For this review, take the finished solid that the model builds, in its own axes (mm). A direction names the side the tool comes from. Give positions to 0.01 mm unless a question says otherwise; leave off trailing zeros. Write each loop counter-clockwise with the first axis right and the second up, starting at its lowest first coordinate (ties: lowest second). Pieces come first, ordered by that corner, then holes. Notation, with made-up numbers: (24.5, -31) -> (42.5, -31) arc R21 ccw to (42.5, -6) -> close; hole circle Ø7 at (56, 6). An arc over 180 degrees is marked (long way). Answer as CSV lines item,"result".
```python
from build123d import *

# Parameters (mm, degrees)
F0_W      = 50.8
F0_H      = 431.8
F1_DEPTH  = 2.54
F2_W      = 2.54
F2_H      = 431.8
F3_DEPTH  = 50.8
F5_DEPTH  = 25.4
F7_DEPTH  = 25.4
F9_DEPTH  = 25.4
F11_DEPTH = 25.4


with BuildPart() as f1:
    # F0 (on Top) → F1 (new body)
    with BuildSketch(Plane.XY):
        with Locations((-30.644535, -61.478847)):
            Rectangle(F0_W, F0_H)
    extrude(amount=F1_DEPTH)

    # F2 (on face) → F3 (join)
    with BuildSketch(Plane(origin=(0, 0, 0), x_dir=(1, 0, 0), z_dir=(0, 0, -1))):
        with Locations((-54.774535, 61.478847)):
            Rectangle(F2_W, F2_H)
    extrude(amount=F3_DEPTH)

    # F4 (on face) → F5 (cut)
    with BuildSketch(Plane(origin=(-56.044535, 0, 0), x_dir=(0, -1, 0), z_dir=(-1, 0, 0))):
        Polygon((277.378847, -50.8), (277.378847, -10.16), (143.720774, -50.8), align=None)
    extrude(amount=-F5_DEPTH, mode=Mode.SUBTRACT)

    # F6 (on face) → F7 (cut)
    with BuildSketch(Plane(origin=(-56.044535, 0, 0), x_dir=(0, -1, 0), z_dir=(-1, 0, 0))):
        Polygon((77.323876, 0), (77.323876, -50.8), (143.720774, -50.8), (277.378847, -10.16), (277.378847, 0), align=None)
    extrude(amount=-F7_DEPTH, mode=Mode.SUBTRACT)

    # F8 (on face) → F9 (cut)
    with BuildSketch(Plane(origin=(-56.044535, 0, 0), x_dir=(0, -1, 0), z_dir=(-1, 0, 0))):
        Polygon((77.323876, -50.8), (77.323876, -45.654178), (71.64523, -50.8), align=None)
    extrude(amount=-F9_DEPTH, mode=Mode.SUBTRACT)

    # F10 (on face) → F11 (cut)
    with BuildSketch(Plane(origin=(-56.044535, 0, 0), x_dir=(0, -1, 0), z_dir=(-1, 0, 0))):
        Polygon((77.323876, -44.246497), (70.091791, -50.8), (71.64523, -50.8), (77.323876, -45.654178), align=None)
    extrude(amount=-F11_DEPTH, mode=Mode.SUBTRACT)


solid = f1.part
```
Q1. Add section B-B (z = -23.5). Write out the cut boundary in (x, y), plus the area to 3 significant figures.
Answer block:
outline,"(-56.04, -77.32) -> (-53.5, -77.32) -> (-53.5, 154.42) -> (-56.04, 154.42) -> close"
area,"589 mm2"
Q2. Clearance check with flat-ended pins moving along their axes: pin 1 (4 mm diameter, centred on x = -43.5, y = -25, fed in from -Z); pin 2 (1 mm diameter, centred on y = 92.5, z = -44.5, fed in from +X); pin 3 (2 mm diameter, centred on x = -55, z = -30, fed in from -Y). State where each tip first meets the part, or that it passes through.
Answer block:
pin 1,"stops at z = 0"
pin 2,"stops at x = -53.5"
pin 3,"stops at y = -77.32"
Q3. Add section A-A (y = 96.5). Write out the cut boundary in (x, z), plus the area to 3 significant figures.
Answer block:
outline,"(-56.04, -50.8) -> (-53.5, -50.8) -> (-53.5, 0) -> (-5.24, 0) -> (-5.24, 2.54) -> (-56.04, 2.54) -> close"
area,"258 mm2"
Q4. For faces 1 (the flat face through (-53.505, 40, -25)), 2 (the flat face through (-31, -58, 2.54)), list the 3-axis set-ups (+Z, -Z, +X, -X, +Y, -Y) from which the entire face can be reached by the end or side of a thin tool; tool diameter is ignored.
Answer block:
face 1,"-Z, +X, +Y, -Y"
face 2,"+Z, +X, -X, +Y, -Y"
Q5. To check wall thickness, follow probe 1 along X at (y, z) = (-18, -1.5); probe 2 along Z at (x, y) = (-34, 6). State the ranges of each line that lie inside material, in increasing order. Write a range as [from, to].
Answer block:
probe 1,"x = [-56.04, -53.5]"
probe 2,"z = [0, 2.54]"
Q6. Add section C-C (x = -31). Write out the cut boundary in (y, z), plus the area to 3 significant figures.
Answer block:
outline,"(-277.38, 0) -> (154.42, 0) -> (154.42, 2.54) -> (-277.38, 2.54) -> close"
area,"1,100 mm2"
